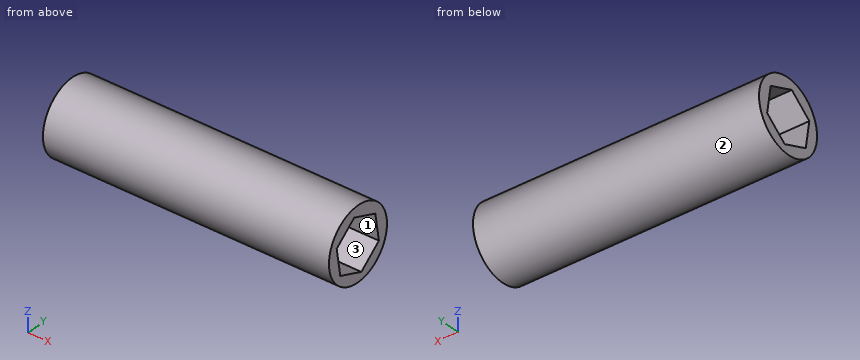
from build123d import *

# Parameters (mm, degrees)
F0_R     = 5.719211
F1_DEPTH = 45
F3_DEPTH = 45.001


with BuildPart() as f1:
    # F0 (on Right) → F1 (new body)
    with BuildSketch(Plane.YZ):
        with Locations((-26.867531, 8.05353)):
            Circle(F0_R)
    extrude(amount=F1_DEPTH)

    # F2 (on Right) → F3 (cut, through all)
    with BuildSketch(Plane.YZ):
        Polygon((-26.200977, 3.548784), (-22.749203, 6.353351), (-23.452142, 10.744959), (-27.606855, 12.332), (-31.058629, 9.527433), (-30.355691, 5.135825), align=None)
    extrude(amount=F3_DEPTH, mode=Mode.SUBTRACT)


solid = f1.part
Work out the finished part from the listing and answer in its coordinate system (mm). Face numbers are marked on the shaded views. Coordinates: 2 decimals unless noted, no trailing zeros. Write each loop counter-clockwise with the first axis right and the second up, starting at its lowest first coordinate (ties: lowest second). Pieces come first, ordered by that corner, then holes. Notation, with made-up numbers: M 79,56 L 101,56 A20 cw 101,62 Z; hole C -12.75,86 d8. An arc over 180 degrees is marked long. Write item = value, one per line.
1. Straight lines are drawn through the part: line 1 (Z direction, x = 19.5, y = -27.5) (3 decimals); line 2 (Y direction, x = 37.5, z = 5.5); line 3 (Y direction, x = 7.5, z = 6). For each, find the intervals that lie inside material, in ascending order. Write a range as from..to.
Solution:
line_1 = 2.369..4.045, 12.291..13.738
line_2 = -31.99..-30.41, -23.8..-21.75
line_3 = -32.21..-30.49, -23.18..-21.53
2. The part is cut by section A-A (y = -24.25). Determine the outline of the cut face in (x, z), then the cut area to 3 significant figures.
Solution:
outline = M 0,2.97 L 45,2.97 L 45,5.13 L 0,5.13 Z; M 0,11.05 L 45,11.05 L 45,13.14 L 0,13.14 Z
area = 191 mm2
3. Determine the mould class of the marked faces 1, 2 and 3 for opening direction Z: released by +Z, released by -Z, zero draft, split by the parting line, or undercut.
Solution:
face_1 = undercut
face_2 = split by the parting line
face_3 = undercut
4. The part is cut by section B-B (z = 11.75). Determine the outline of the cut face in (x, y), then the cut area to 3 significant figures.
Solution:
outline = M 0,-31.23 L 45,-31.23 L 45,-28.32 L 0,-28.32 Z; M 0,-26.08 L 45,-26.08 L 45,-22.5 L 0,-22.5 Z
area = 292 mm2
5. The part is cut by section C-C (x = 24). Determine the outline of the cut face in (y, z), then the cut area to 3 significant figures.
Solution:
outline = C -26.87,8.05 d11.44; hole M -31.06,9.53 L -30.36,5.14 L -26.2,3.55 L -22.75,6.35 L -23.45,10.74 L -27.61,12.33 Z
area = 51.4 mm2
6. Flat-ended cylindrical pins translate along their axes: pin 1 (6 mm diameter, centred on x = 37.5, z = 3.5, fed in from -Y); pin 2 (2 mm diameter, centred on x = 39.5, y = -23.5, fed in from +Z); pin 3 (4 mm diameter, centred on x = 32.5, y = -27.5, fed in from +Z). Find the tip coordinate at first contact, or state that the pin passes through.
Solution:
pin_1 = -32.37
pin_2 = 13.26
pin_3 = 13.77
7. The part is cut by section D-D (y = -22.25). Determine the outline of the cut face in (x, z).
Solution:
outline = M 0,4.68 L 45,4.68 L 45,11.43 L 0,11.43 Z
